from build123d import *

# Parameters (mm, degrees)
F2_W            = 4
F2_H            = 8
F3_DEPTH        = 25
F5_DEPTH        = 28.501
F5_COPIES_COUNT = 3


# Not quite as in the source:
# - a pattern or mirror of a feature is missing from the dataset's text; its kind, count and spacing are read off the source's solid


with BuildPart() as f1:
    # F0 (on Front) → F1 (revolve)
    with BuildSketch(Plane.XZ):
        Polygon((0, 11), (0, 6), (17, 6), (17, 15), (28.5, 37.5), (28.5, 49.25), (18, 49.25), (18, 37.5), (10, 15), (10, 11), align=None)
    revolve(axis=Axis((-9.663007474, 0, 0), (-1, 0, 0)))

    # F2 (on Right) → F3 (cut)
    with BuildSketch(Plane.YZ):
        with Locations((0, 4)):
            Rectangle(F2_W, F2_H)
    extrude(amount=F3_DEPTH, mode=Mode.SUBTRACT)

    # F4 (on face) → F5 (cut, through all)
    with BuildSketch(Plane.YZ.offset(28.5)):
        with BuildLine():
            Line((7.5, 12.9903810568), (29.0575654097, 23.7045964416))
            ThreePointArc((29.0575654097, 23.7045964416), (0, 37.5), (-29.0575654097, 23.7045964416))
            Line((-29.0575654097, 23.7045964416), (-7.5, 12.9903810568))
            ThreePointArc((-7.5, 12.9903810568), (0, 15), (7.5, 12.9903810568))
        make_face()
    f5 = extrude(amount=-F5_DEPTH, mode=Mode.SUBTRACT)

    # F5_copies: F5 ×3 about axis
    f5_copies_axis = Axis((0, 0, 0), (1, 0, 0))
    for i in range(1, F5_COPIES_COUNT):
        add(f5.rotate(f5_copies_axis, i * 360 / F5_COPIES_COUNT), mode=Mode.SUBTRACT)


solid = f1.part
Geometry: final body of the model. Coordinates: model frame, mm. A direction names the side the tool comes from. Round coordinates to 2 decimals unless told otherwise and drop trailing zeros. Loops run counter-clockwise (first coordinate to the right, second up) from the corner with the lowest first, then second, coordinate; pieces in that order, holes last.
Q1. Material intervals for L1, parallel to Y at x = 5.25, z = 0; L2, parallel to X at y = -37.5, z = -20; L3, parallel to Y at x = 22.5, z = 24, sorted ascending.
Q2. Access query for faces 4 (the conical face through (21.55, -20.79, 11.8)), 5 (the flat face through (19.38, -24.888, 6.563)), 6 (the conical face through (13.055, 20.345, 11.946)), 7 (the flat face through (18, -36.3, -11.2)). Directions: +Z, -Z, +X, -X, +Y, -Y. A direction counts if a zero-diameter tool reaches every point of the face in a straight line with its end or side. Return the directions, or none.
Q3. Pin query (flat end, axial travel): P1, Ø4, axis at y = -9, z = 12, coming from the +X side; P2, Ø4, axis at x = 18.5, y = 36.5, coming from the -Z side; P3, Ø1.5, axis at x = 11, z = -17.5, coming from the -Y side. Return the tip coordinate at first contact, or that it passes through.
Q4. Section D-D on x = 21. Return loops of the section in (y, z).
Q5. Section C-C on z = 34. Return loops of the section in (x, y).
Q6. Section A-A on y = 0. Return loops of the section in (x, z), plus the area to 3 significant figures.
Q7. Pull-direction query (Z, two-part tool) for faces 1 (the cylindrical face through (13.549, -12.935, -7.595)), 2 (the cylindrical face through (23.324, 0.465, 37.497)), 3 (the flat face through (17, 0.2, -6.5)); classes: released by +Z, released by -Z, zero draft, split by the parting line, or undercut.
Q8. Section B-B on x = 6.5. Return loops of the section in (y, z).
Evaluation:
1. L1: y = -11 to -6, 6 to 11
1. L2: x = 18 to 28.5
1. L3: y = -43.01 to -28.81, 28.81 to 43.01
2. face 4: +X
2. face 5: +X, -X
2. face 6: +Z, -X, +Y
2. face 7: -X
3. P1: stops at x = 18.02
3. P2: stops at z = -35.15
3. P3: stops at y = -7.26
4. outline: circle Ø98.5 at (0, 0); hole (-35.06, 13.31) arc R37.5 ccw to (-6, -37.02) - (-6.95, -21.74) arc R22.83 ccw to (6.95, -21.74) - (6, -37.02) arc R37.5 ccw to (35.06, 13.31) - (22.31, 4.85) arc R22.83 ccw to (15.35, 16.89) - (29.06, 23.7) arc R37.5 ccw to (-29.06, 23.7) - (-15.35, 16.89) arc R22.83 ccw to (-22.31, 4.85) - close
5. outline: (18, -35.63) - (28.5, -35.63) - (28.5, -15.82) - (18, -15.82) - close; (18, 15.82) - (28.5, 15.82) - (28.5, 35.63) - (18, 35.63) - close
6. outline: (0, -11) - (10, -11) - (10, -15) - (18, -37.5) - (18, -49.25) - (28.5, -49.25) - (28.5, -37.5) - (17, -15) - (17, -6) - (0, -6) - close; (0, 8) - (17, 8) - (17, 15) - (10, 15) - (10, 11) - (0, 11) - close; (18, 37.5) - (28.5, 37.5) - (28.5, 49.25) - (18, 49.25) - close
6. area: 636 mm2
7. face 1: released by -Z
7. face 2: undercut
7. face 3: zero draft
8. outline: circle Ø22 at (0, 0); hole (-2, 5.66) arc R6 ccw (long way) to (2, 5.66) - (2, 8) - (-2, 8) - close
